Can you work these out from the model? Positions are in its coordinate system, mm. A direction names the side the tool comes from. Coordinates: 2 decimals unless noted, no trailing zeros. Order: outer loops, then holes, each group sorted by start corner. A loop starts at its lowest first (then second) coordinate and runs counter-clockwise, first axis right, second up.
```python
from build123d import *

# Parameters (mm, degrees)
F0_R     = 2.5
F1_DEPTH = 25
F2_DEPTH = 5
F3_R     = 3


with BuildPart() as f1:
    # F0 (on Top) → F1 (new body)
    with BuildSketch(Plane.XY):
        with BuildLine():
            Line((-48.6113993327, 56.4697863751), (-50.6071856175, 56.6486881103))
            ThreePointArc((-50.6071856175, 56.6486881103), (-60.4968157511, 46.7759208686), (-50.8603799334, 36.6558703788))
            Line((-50.8603799334, 36.6558703788), (-46.6194621468, 37.431918344))
            ThreePointArc((-46.6194621468, 37.431918344), (-42.1675049005, 41.1167281405), (-40.4976175725, 46.6492883861))
            ThreePointArc((-40.4976175725, 46.6492883861), (-42.7884612504, 53.0186611025), (-48.6113993327, 56.4697863751))
        make_face()
        with Locations((-50.4976175725, 46.6492883861)):
            Circle(F0_R, mode=Mode.SUBTRACT)
    extrude(amount=F1_DEPTH)

    # F0 (on Top) → F2 (join)
    with BuildSketch(Plane.XY):
        with BuildLine():
            Line((-48.6113993327, 56.4697863751), (-50.6071856175, 56.6486881103))
            ThreePointArc((-50.6071856175, 56.6486881103), (-60.4968157511, 46.7759208686), (-50.8603799334, 36.6558703788))
            Line((-50.8603799334, 36.6558703788), (-46.6194621468, 37.431918344))
            ThreePointArc((-46.6194621468, 37.431918344), (-42.1675049005, 41.1167281405), (-40.4976175725, 46.6492883861))
            ThreePointArc((-40.4976175725, 46.6492883861), (-42.7884612504, 53.0186611025), (-48.6113993327, 56.4697863751))
        make_face()
        with Locations((-50.4976175725, 46.6492883861)):
            Circle(F0_R, mode=Mode.SUBTRACT)
        with BuildLine():
            ThreePointArc((-48.6113993327, 56.4697863751), (-49.6048001576, 56.6093524955), (-50.6071856175, 56.6486881103))
            Line((-50.6071856175, 56.6486881103), (-48.6113993327, 56.4697863751))
        make_face()
        with BuildLine():
            Line((-46.6194621468, 37.431918344), (-50.8603799334, 36.6558703788))
            ThreePointArc((-50.8603799334, 36.6558703788), (-48.6976009861, 36.8126253194), (-46.6194621468, 37.431918344))
        make_face()
        with BuildLine():
            Line((0, 52.1122738719), (-48.6113993327, 56.4697863751))
            ThreePointArc((-48.6113993327, 56.4697863751), (-42.7884612504, 53.0186611025), (-40.4976175725, 46.6492883861))
            ThreePointArc((-40.4976175725, 46.6492883861), (-42.1675049005, 41.1167281405), (-46.6194621468, 37.431918344))
            Line((-46.6194621468, 37.431918344), (0, 45.9628403187))
            Line((0, 45.9628403187), (0, 52.1122738719))
        make_face()
    extrude(amount=F2_DEPTH)

    # F3
    f3_edges = [f1.edges().sort_by_distance(p)[0] for p in [
        (0, 45.96284, 2.5),
        (0, 52.112274, 2.5),
        (-23.309731, 41.697379, 0),
        (-24.3057, 54.29103, 0),
    ]]
    fillet(f3_edges, radius=F3_R)


solid = f1.part
```
1. I'm going to push flat-ended pins straight in: pin 1 (2 mm diameter, centred on x = -42, z = 15.5, fed in from +Y); pin 2 (2 mm diameter, centred on x = -37.5, z = 5, fed in from +Y); pin 3 (9.5 mm diameter, centred on x = -16, y = 49, fed in from +Z). Where does each tip first touch, or does it pass through?
Completed:
pin 1: stops at y = 53.27
pin 2: stops at y = 55.56
pin 3: stops at z = 5
2. Imagine slicing it at A-A on z = 19.75. Please give me the cut outline in (x, y).
Completed:
outline: (-50.86, 36.66) - (-46.62, 37.43) arc R10 ccw to (-48.61, 56.47) - (-50.61, 56.65) arc R10 ccw to start; hole circle Ø5 at (-50.5, 46.65)
3. Thinking about a two-plate mould opening in Y: for faces 1 (the cylindrical face through (-50.82, 49.13, 12.32)), 2 (the cylindrical face through (-22.86, 42.65, 0.9)), 3 (the flat face through (-48, 45, 25)), which applies, pulls with the +Y half, pulls with the -Y half, needs draft (parallel to the pull), parting line crosses it, or undercut?
Completed:
face 1: undercut
face 2: pulls with the -Y half
face 3: needs draft
4. Please list where these lines run through material, in increasing order: probe 1 along Z at (x, y) = (-33, 42.5); probe 2 along Y at (x, z) = (-48.5, 11.75); probe 3 along X at (y, z) = (47.5, 8.5).
Completed:
probe 1: z = 0.04 to 5
probe 2: y = 37.09 to 45.15, 48.15 to 56.45
probe 3: x = -60.46 to -52.85, -48.15 to -40.53
5. On a 3-axis mill with a long thin cutter (end or side, diameter ignored), from which of +Z, -Z, +X, -X, +Y, -Y can I reach the whole of each face in a straight line? I mean faces 4 (the cylindrical face through (-24.594, 53.411, 0.855)), 5 (the flat face through (-48.77, 37.04, 14.86)), 6 (the flat face through (-49.6, 56.56, 14.86)). Say none if no direction works.
Completed:
face 4: -Z, +X, +Y
face 5: +Z, +X, -Y
face 6: +Z, +X, +Y
